For this review, take the finished solid that the model builds, in its own axes (mm). A direction names the side the tool comes from. Round coordinates to 2 decimals unless told otherwise and drop trailing zeros. Order: outer loops, then holes, each group sorted by start corner. A loop starts at its lowest first (then second) coordinate and runs counter-clockwise, first axis right, second up. Notation, with made-up numbers: M -1,-9.75 L 42,-9.75 A19 cw 42,19.25 Z; hole C 13,61 d8. An arc over 180 degrees is marked long. Answer in a Markdown table with one row per item. Add a question column.
```python
from build123d import *

# Parameters (mm, degrees)
F0_W     = 60
F0_H     = 22
F0_R     = 2.125
F0_R_2   = 8.225
F1_DEPTH = 27
F2_DEPTH = 21
F3_R     = 3.25
F4_DEPTH = 22.001
F5_DEPTH = 24.35
F6_R     = 5.9
F7_DEPTH = 27.001


with BuildPart() as f1:
    # F0 (on Front) → F1 (new body)
    with BuildSketch(Plane.XZ):
        Rectangle(F0_W, F0_H)
        with Locations((-12.6, 0)):
            Circle(F0_R, mode=Mode.SUBTRACT)
        Circle(F0_R_2, mode=Mode.SUBTRACT)
        with Locations((12.6, 0)):
            Circle(F0_R, mode=Mode.SUBTRACT)
        Circle(F0_R_2)
        with Locations((-12.6, 0)):
            Circle(F0_R)
        with Locations((12.6, 0)):
            Circle(F0_R)
    extrude(amount=F1_DEPTH)

    # F0 (on Front) → F2 (cut)
    with BuildSketch(Plane.XZ):
        with Locations((12.6, 0)):
            Circle(F0_R)
        with Locations((-12.6, 0)):
            Circle(F0_R)
    extrude(amount=F2_DEPTH, mode=Mode.SUBTRACT)

    # F3 (on face) → F4 (cut, through all)
    with BuildSketch(Plane.XY.offset(11)):
        with Locations((22.25, -19.25)):
            Circle(F3_R)
        with Locations((-22.25, -19.25)):
            Circle(F3_R)
    extrude(amount=-F4_DEPTH, mode=Mode.SUBTRACT)

    # F0 (on Front) → F5 (cut)
    with BuildSketch(Plane.XZ):
        Circle(F0_R_2)
    extrude(amount=F5_DEPTH, mode=Mode.SUBTRACT)

    # F6 (on face) → F7 (cut, through all)
    with BuildSketch(Plane.XZ.offset(27)):
        Circle(F6_R)
    extrude(amount=-F7_DEPTH, mode=Mode.SUBTRACT)


solid = f1.part
```
1. To check wall thickness, follow probe 1 along Z at (x, y) = (0, -9.25) (3 decimals); probe 2 along Z at (x, y) = (0, -25.9); probe 3 along X at (y, z) = (-18.5, -0.25). State the ranges of each line that lie inside material, in increasing order. Write a range as [from, to].
2. Consider section D-D on x = 12.6. Write out the cut boundary in (y, z) (3 decimals), plus the area to 3 significant figures.
3. For faces 5 (the flat face through (-13, -21, 0)), 6 (the flat face through (-7, 0, 5)), list the 3-axis set-ups (+Z, -Z, +X, -X, +Y, -Y) from which the entire face can be reached by the end or side of a thin tool; tool diameter is ignored.
4. Consider section C-C on y = -9.25. Write out the cut boundary in (x, z) (3 decimals), plus the area to 3 significant figures.
5. Consider section A-A on z = 0. Write out the cut boundary in (x, y) (3 decimals), plus the area to 3 significant figures.
6. Clearance check with a flat-ended pin moving along its axis: pin 1 Ø4 at (x, z) = (12.6, 0) entering from +Y. State where the tip first meets the part, or that it passes through.
7. The part is to be moulded in two halves that separate along Z. For faces 1 (the flat face through (0, -13, -11)), 2 (the flat face through (-30, -13, 0)), 3 (the flat face through (0, -13, 11)), 4 (the cylindrical face through (-1.78, -12, -8.03)), say which applies: pulls with the +Z half, pulls with the -Z half, needs draft (parallel to the pull), parting line crosses it, or undercut.
8. Consider section B-B on x = -22.25. Write out the cut boundary in (y, z), plus the area to 3 significant figures.
Solved:
| question | item | result |
|---|---|---|
| 1 | probe 1 | z = [-11, -8.225], [8.225, 11] |
| 1 | probe 2 | z = [-11, -5.9], [5.9, 11] |
| 1 | probe 3 | x = [-30, -25.41], [-19.09, -14.71], [-10.49, -8.22], [8.22, 10.49], [14.71, 19.09], [25.41, 30] |
| 2 | outline | M -27,-11 L 0,-11 L 0,-2.125 L -21,-2.125 L -21,2.125 L 0,2.125 L 0,11 L -27,11 Z |
| 2 | area | 505 mm^2 |
| 3 | face 5 | +Y |
| 3 | face 6 | +Z, -Z, +X, -X, +Y |
| 4 | outline | M -30,-11 L 30,-11 L 30,11 L -30,11 Z; hole C -12.6,0 d4.25; hole C 0,0 d16.45; hole C 12.6,0 d4.25 |
| 4 | area | 1,080 mm^2 |
| 5 | outline | M -30,-27 L -5.9,-27 L -5.9,-24.35 L -8.225,-24.35 L -8.225,0 L -10.475,0 L -10.475,-21 L -14.725,-21 L -14.725,0 L -30,0 Z; M 5.9,-27 L 30,-27 L 30,0 L 14.725,0 L 14.725,-21 L 10.475,-21 L 10.475,0 L 8.225,0 L 8.225,-24.35 L 5.9,-24.35 Z; hole C -22.25,-19.25 d6.5; hole C 22.25,-19.25 d6.5 |
| 5 | area | 943 mm^2 |
| 6 | pin 1 | stops at y = -21 |
| 7 | face 1 | pulls with the -Z half |
| 7 | face 2 | needs draft |
| 7 | face 3 | pulls with the +Z half |
| 7 | face 4 | undercut |
| 8 | outline | M -27,-11 L -22.5,-11 L -22.5,11 L -27,11 Z; M -16,-11 L 0,-11 L 0,11 L -16,11 Z |
| 8 | area | 451 mm^2 |
